Could you check a few things on this model? Use its own coordinates, in mm. A direction names the side the tool comes from. Coordinates: 2 decimals unless noted, no trailing zeros. Write each loop counter-clockwise with the first axis right and the second up, starting at its lowest first coordinate (ties: lowest second). Pieces come first, ordered by that corner, then holes.
Autodesk Inventor part; units mm, degrees
ref_plane "YZ Plane" through (0, 0, 0) normal (1, 0, 0) x (0, 1, 0)
ref_plane "XZ Plane" through (0, 0, 0) normal (0, 1, 0) x (-1, 0, 0)
ref_plane "XY Plane" through (0, 0, 0) normal (0, 0, 1) x (1, 0, 0)
sketch "Náčrt1" plane through (0, 0, 0) normal (0, 0, 1) x (1, 0, 0)
  line L0 (13.97, 23.865) -> (13.97, 9.144)
  line L1 (0, 9.144) -> (0, 0)
  line L2 (4.5409, 9.144) -> (0, 9.144)
  line L3 (4.5409, 8.255) -> (4.5409, 9.144)
  line L4 (3.2709, 6.985) -> (4.5409, 8.255)
  line L5 (3.2709, 4.318) -> (3.2709, 6.985)
  line L6 (8.7319, 9.144) -> (8.7319, 8.255)
  line L7 (13.97, 9.144) -> (8.7319, 9.144)
  line L8 (8.7319, 8.255) -> (10.0019, 6.985)
  line L9 (10.0019, 6.985) -> (10.0019, 4.318)
  line L10 (10.0019, 4.318) -> (3.2709, 4.318)
  line L11 (0, 0) -> (19.97, 0)
  line L12 (13.97, 22.5956) -> (13.97, 25.1349)
  line L13 (13.97, 20.4353) -> (13.97, 18.035)
  line L14 (13.97, 25.1349) -> (19.97, 25.1349)
  line L15 (19.97, 25.1349) -> (19.97, 0)
extrude "Vysunutí1" add sketch "Náčrt1" against normal blind 32.6
sketch "Náčrt2" plane through (19.97, 0, 0) normal (1, 0, 0) x (0, 0, -1)
  line L0 (0, 25.1349) -> (32.6, 25.1349)
  line L1 (16.3, 25.1349) -> (4.746, 25.1349)
  line L2 (4.746, 25.1349) -> (4.746, 12.9539)
  line L3 (16.3, 25.1349) -> (27.854, 25.1349)
  line L4 (27.854, 25.1349) -> (27.854, 12.9539)
  line L5 (27.854, 12.9539) -> (4.746, 12.9539)
  circle A0 centre (2.8, 19.2349) radius 1.2
  line L6 (16.3, 25.1349) -> (16.3, 15.9225)
  circle A1 centre (29.8, 19.2349) radius 1.2
  point P0 (0, 0)
  point P1 (4.746, 19.0444)
  dimension "d2" = 11.554
  dimension "d3" = 12.181
  dimension "d4" = 11.554
  dimension "d7" = 2.4
  dimension "d8" = 5.9
  dimension "d9" = 1.946
extrude "Vysunutí2" cut sketch "Náčrt2" against normal blind 32.6 contours L0 L4 L5 L2
extrude "Vysunutí3" cut sketch "Náčrt2" against normal blind 32.6 contours A0 | A1
fillet "Zaoblení1" radius 2 4 edges at (16.97, 25.1349, 0) (16.97, 25.1349, -4.746) (16.97, 25.1349, -27.854) (16.97, 25.1349, -32.6)
sketch "Náčrt3" plane through (0, 0, 0) normal (0, -1, 0) x (1, 0, 0)
  point P0 (0, 0)
sketch "Náčrt4" plane through (0, 0, 0) normal (0, 0, 1) x (1, 0, 0)
  line L0 (13.97, 23.1349) -> (19.97, 23.1349)
  line L1 (13.97, 23.1349) -> (13.97, 9.144)
  line L2 (13.97, 9.144) -> (8.7319, 9.144)
  line L3 (8.7319, 9.144) -> (8.7319, 8.255)
  line L4 (8.7319, 8.255) -> (10.0019, 6.985)
  line L5 (10.0019, 6.985) -> (10.0019, 4.318)
  line L6 (10.0019, 4.318) -> (3.2709, 4.318)
  line L7 (3.2709, 4.318) -> (3.2709, 6.985)
  line L8 (3.2709, 6.985) -> (4.5409, 8.255)
  line L9 (4.5409, 8.255) -> (4.5409, 9.144)
  line L10 (4.5409, 9.144) -> (0, 9.144)
  line L11 (0, 9.144) -> (0, 0)
  line L12 (0, 0) -> (19.97, 0)
  line L13 (19.97, 0) -> (19.97, 23.1349)
  line L14 (0, 0) -> (-8, 0)
  line L15 (-8, 0) -> (-8, 14)
  line L16 (-8, 14) -> (0, 14)
  line L17 (0, 14) -> (0, 0)
  dimension "d13" = 14
  dimension "d14" = 8
extrude "Vysunutí4" add sketch "Náčrt4" along normal blind 12 and the other way blind 32.6 contours L14 L15 L16 L17 L11
sketch "Náčrt5" plane through (0, 0, 0) normal (1, 0, 0) x (0, 0, -1)
  line L0 (0, 9.144) -> (0, 0)
  line L1 (0, 9.144) -> (32.6, 9.144)
  line L2 (32.6, 14) -> (32.6, 9.144)
  line L3 (32.6, 14) -> (-12, 14)
  line L4 (-12, 0) -> (-12, 14)
  line L5 (0, 0) -> (-12, 0)
  circle A0 centre (-6.5, 7) radius 2.25
  line L6 (27.854, 12.9539) -> (4.746, 12.9539)
  line L7 (16.3, 12.9539) -> (16.3, -5.3216)
  line L8 (32.6, 9.144) -> (32.6, 0)
  line L9 (44.6, 0) -> (44.6, 14)
  line L10 (32.6, 0) -> (44.6, 0)
  circle A1 centre (39.1, 7) radius 2.25
  line L11 (44.6, 14) -> (32.6, 14)
  line L12 (32.6, 14) -> (32.6, 0)
  dimension "d19" = 4.5
  dimension "d20" = 7
  dimension "d21" = 5.5
extrude "Vysunutí5" add sketch "Náčrt5" against normal up to surface (8 mm away) contours L2 L11 L9 L10 L8 | A0
sketch "Náčrt6" plane through (0, 0, 12) normal (0, 0, 1) x (1, 0, 0)
  line L0 (-8, 14) -> (-8, 0)
  line L1 (-8, 0) -> (0, 0)
  line L2 (0, 0) -> (0, 14)
  line L3 (0, 14) -> (-8, 14)
  line L4 (0, 14) -> (-4, 14)
  line L5 (-4, 14) -> (-4, 0)
  line L6 (-4, 0) -> (0, 0)
  line L7 (0, 0) -> (0, 14)
  dimension "d24" = 4
extrude "Vysunutí6" cut sketch "Náčrt6" against normal blind 12 contours L3 L2 L1 L5
extrude "Vysunutí7" cut sketch "Náčrt5" against normal blind 4 contours L2 L11 L9 L10 L8
sketch "Náčrt7" plane through (0, 0, 12) normal (0, 0, 1) x (1, 0, 0)
  line L0 (-4, 0) -> (-4, 14)
  line L1 (-4, 14) -> (-8, 14)
  line L2 (-8, 14) -> (-8, 0)
  line L3 (-8, 0) -> (-4, 0)
  point P0 (0, 0)
extrude "Vysunutí8" cut sketch "Náčrt7" against normal up to surface (12 mm away)
properties part number "Motor_holder" material "Měď"
1. Please list where these lines run through material, in increasing order: line 1 along X through (y, z) = (4.5, -13); line 2 along Z through (x, y) = (15.5, 17.25); line 3 along X through (y, z) = (12.5, -24).
Verdict:
line 1: x = -8 to 3.27, 10 to 19.97
line 2: z = -32.6 to -27.85, -4.75 to 0
line 3: x = -8 to 0, 13.97 to 19.97
2. I want a section at C-C on x = 14.75. Please give me the cut outline in (y, z).
Verdict:
outline: (0, -32.6) - (23.13, -32.6) arc R2 ccw to (25.13, -30.6) - (25.13, -29.85) arc R2 ccw to (23.13, -27.85) - (12.95, -27.85) - (12.95, -4.75) - (23.13, -4.75) arc R2 ccw to (25.13, -2.75) - (25.13, -2) arc R2 ccw to (23.13, 0) - (0, 0) - close; hole circle Ø2.4 at (19.23, -29.8); hole circle Ø2.4 at (19.23, -2.8)
3. I want a section at D-D on z = -14. Please give me the cut outline in (x, y) (3 decimals), plus the area to 3 significant figures.
Verdict:
outline: (-8, 0) - (19.97, 0) - (19.97, 12.954) - (13.97, 12.954) - (13.97, 9.144) - (8.732, 9.144) - (8.732, 8.255) - (10.002, 6.985) - (10.002, 4.318) - (3.271, 4.318) - (3.271, 6.985) - (4.541, 8.255) - (4.541, 9.144) - (0, 9.144) - (0, 14) - (-8, 14) - close
area: 289 mm2
4. I want a section at A-A on y = 14.75. Please give me the cut outline in (x, z), plus the area to 3 significant figures.
Verdict:
outline: (13.97, -32.6) - (19.97, -32.6) - (19.97, -27.85) - (13.97, -27.85) - close; (13.97, -4.75) - (19.97, -4.75) - (19.97, 0) - (13.97, 0) - close
area: 57.0 mm2
5. For pin 1 (12 mm diameter, centred on x = -2, z = -16.5, fed in from +Y); pin 2 (1.5 mm diameter, centred on x = 15, y = 21, fed in from -Z); pin 3 (5 mm diameter, centred on x = 13, z = -25, fed in from +Y); pin 4 (5 mm diameter, centred on y = 18.5, z = -11.5, fed in from -X), each with a flat end and sliding along its axis, tell me the tip position at first contact or that it passes through.
Verdict:
pin 1: stops at y = 14
pin 2: stops at z = -32.6
pin 3: stops at y = 12.95
pin 4: passes through
6. If we mould it in two halves opening along Y, with no side actions, what happens to faces 1 (the face through (-5.972, 7.099, -36.852)), 2 (the face through (-4, 5.5, -37.2)), 3 (the face through (7, 4.318, -16)), 4 (the face through (17.012, 24.533, -32.03))? For each: pulls with the +Y half, pulls with the -Y half, needs draft (parallel to the pull), parting line crosses it, or undercut.
Verdict:
face 1: undercut
face 2: needs draft
face 3: undercut
face 4: pulls with the +Y half
7. I want a section at B-B on z = -39.1. Please give me the cut outline in (x, y).
Verdict:
outline: (-8, 0) - (-4, 0) - (-4, 4.75) - (-8, 4.75) - close; (-8, 9.25) - (-4, 9.25) - (-4, 14) - (-8, 14) - close
8. On a 3-axis mill with a long thin cutter (end or side, diameter ignored), from which of +Z, -Z, +X, -X, +Y, -Y can I reach the whole of each face in a straight line? I mean faces 5 (the face through (17, 19.3, -28.6)), 6 (the face through (0, 12, -17)), 7 (the face through (10.002, 6, -16)). Say none if no direction works.
Verdict:
face 5: +X, -X
face 6: +Z, -Z, +Y
face 7: +Z, -Z
